CAD build for the part. Positions are in the model's coordinates, mm. Round coordinates to 2 decimals unless told otherwise and drop trailing zeros. Loops run counter-clockwise (first coordinate to the right, second up) from the corner with the lowest first, then second, coordinate; pieces in that order, holes last. Notation, with made-up numbers: M 89,-35 L 116,-35 A25 ccw 116,-15 Z; hole C 63,41.5 d6. An arc over 180 degrees is marked long. Put each result on its own line as item: value. Start each with the question number.
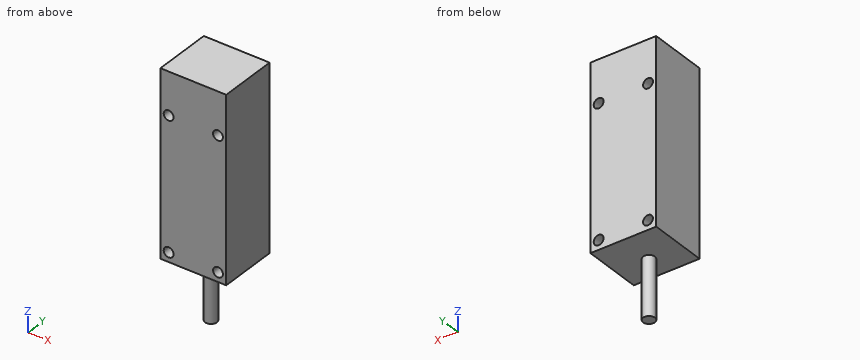
from build123d import *

# Parameters (mm, degrees)
SKETCH1_W           = 28
SKETCH1_H           = 25
BOSS_EXTRUDE1_DEPTH = 39
SKETCH2_R           = 2.1
CUT_EXTRUDE1_DEPTH  = 49.39421453
SKETCH3_R           = 2.5
BOSS_EXTRUDE2_DEPTH = 25


with BuildPart() as part:
    # Sketch1 → Boss-Extrude1 (new, symmetric)
    with BuildSketch(Plane.XY):
        Rectangle(SKETCH1_W, SKETCH1_H)
    extrude(amount=BOSS_EXTRUDE1_DEPTH, both=True)

    # Sketch2 → Cut-Extrude1 (cut, through all)
    with BuildSketch(Plane(origin=(0, 12.5, 0), x_dir=(1, 0, 0), z_dir=(0, 1, 0))):
        with Locations(Location((10.5, 35, 0), (0, 0, 180))):
            Circle(SKETCH2_R)
        with Locations(Location((10.5, -21, 0), (0, 0, 180))):
            Circle(SKETCH2_R)
    cut_extrude1 = extrude(amount=-CUT_EXTRUDE1_DEPTH, mode=Mode.SUBTRACT)

    # Mirror1: Cut-Extrude1 across plane
    add(cut_extrude1.mirror(Plane(origin=(0, 0, 0), x_dir=(0, 0, 1), z_dir=(1, 0, 0))), mode=Mode.SUBTRACT)

    # Sketch3 → Boss-Extrude2 (add)
    with BuildSketch(Plane(origin=(0, 0, -39), x_dir=(-1, 0, 0), z_dir=(0, 0, -1))):
        with Locations(Location((0, -2.3, 0), (0, 0, 180))):
            Circle(SKETCH3_R)
    extrude(amount=BOSS_EXTRUDE2_DEPTH)


solid = part.part
(1) Cut at C-C on y = 8.75. List the corners of the cut face in (x, z), and give its area (3 significant figures).
(2) Flat gauge pins, fed straight in: pin 1 Ø10 at (x, y) = (-8, -0.5) entering from -Z; pin 2 Ø2.5 at (x, z) = (-10.5, 21) entering from -Y. Where does each tip first touch, or does it go through?
(3) Cut at B-B on x = 10.5. List the corners of the cut face in (y, z).
(4) Cut at D-D on x = 0. List the corners of the cut face in (y, z), and give its area (4 significant figures).
(5) Drill centre lines: line 1 along Z through (x, y) = (10.5, 4.25); line 2 along X through (y, z) = (-10.25, 19.5); line 3 along Z through (x, y) = (-11, 2.25). Where is each one in solid material? Low to high.
(6) Cut at A-A on z = 21. List the corners of the cut face in (x, y).
Taken from the geometry:
1. outline: M -14,-39 L 14,-39 L 14,39 L -14,39 Z; hole C -10.5,-35 d4.2; hole C -10.5,21 d4.2; hole C 10.5,-35 d4.2; hole C 10.5,21 d4.2
1. area: 2,130 mm2
2. pin 1: z = -39
2. pin 2: through
3. outline: M -12.5,-39 L 12.5,-39 L 12.5,-37.1 L -12.5,-37.1 Z; M -12.5,-32.9 L 12.5,-32.9 L 12.5,18.9 L -12.5,18.9 Z; M -12.5,23.1 L 12.5,23.1 L 12.5,39 L -12.5,39 Z
4. outline: M -12.5,-39 L -4.8,-39 L -4.8,-64 L 0.2,-64 L 0.2,-39 L 12.5,-39 L 12.5,39 L -12.5,39 Z
4. area: 2,075 mm2
5. line 1: -39 to -37.1, -32.9 to 18.9, 23.1 to 39
5. line 2: -14 to -11.97, -9.03 to 9.03, 11.97 to 14
5. line 3: -39 to -37.04, -32.96 to 18.96, 23.04 to 39
6. outline: M -14,-12.5 L -12.6,-12.5 L -12.6,12.5 L -14,12.5 Z; M -8.4,-12.5 L 8.4,-12.5 L 8.4,12.5 L -8.4,12.5 Z; M 12.6,-12.5 L 14,-12.5 L 14,12.5 L 12.6,12.5 Z
